```python
from build123d import *

# Parameters (mm, degrees)
F0_W      = 600
F0_H      = 600
F1_DEPTH  = 100
F3_R      = 2
F4_T      = -1.6
F6_DEPTH  = 100.001
F8_DEPTH  = 100.001
F9_R      = 4
F10_DEPTH = 100.001


with BuildPart() as f1:
    # F0 (on Top) → F1 (new body)
    with BuildSketch(Plane.XY):
        Rectangle(F0_W, F0_H)
    extrude(amount=F1_DEPTH)

    # F3
    f3_edges = [f1.edges().sort_by_distance(p)[0] for p in [
        (0, -300, 100),
        (-300, -300, 50),
        (-300, 0, 100),
        (300, -300, 50),
        (-300, 300, 50),
        (300, 0, 100),
        (0, 300, 100),
        (300, 300, 50),
    ]]
    fillet(f3_edges, radius=F3_R)

    # F4
    f4_openings = [f1.faces().sort_by_distance(p)[0] for p in [
        (0, 0, 0),
    ]]
    offset(amount=F4_T, openings=f4_openings)

    # F5 (on face) → F6 (cut, through all)
    with BuildSketch(Plane.XY.offset(100)):
        with BuildLine():
            Line((298, 300), (298, 298))
            Line((298, 298), (300, 298))
            ThreePointArc((300, 298), (299.414214, 299.414214), (298, 300))
        make_face()
        with BuildLine():
            Line((298, -298), (298, -300))
            ThreePointArc((298, -300), (299.414214, -299.414214), (300, -298))
            Line((300, -298), (298, -298))
        make_face()
        with BuildLine():
            Line((-300, 298), (-298, 298))
            Line((-298, 298), (-298, 300))
            ThreePointArc((-298, 300), (-299.414214, 299.414214), (-300, 298))
        make_face()
        with BuildLine():
            ThreePointArc((-300, -298), (-299.414214, -299.414214), (-298, -300))
            Line((-298, -300), (-298, -298))
            Line((-298, -298), (-300, -298))
        make_face()
    extrude(amount=-F6_DEPTH, mode=Mode.SUBTRACT)

    # F7 (on face) → F8 (cut, through all)
    with BuildSketch(Plane.XY.offset(100)):
        with BuildLine():
            ThreePointArc((-20.5, -9.5), (-17.278175, -17.278175), (-9.5, -20.5))
            Line((-9.5, -20.5), (9.5, -20.5))
            ThreePointArc((9.5, -20.5), (17.278175, -17.278175), (20.5, -9.5))
            Line((20.5, -9.5), (20.5, 9.5))
            ThreePointArc((20.5, 9.5), (17.278175, 17.278175), (9.5, 20.5))
            Line((9.5, 20.5), (-9.5, 20.5))
            ThreePointArc((-9.5, 20.5), (-17.278175, 17.278175), (-20.5, 9.5))
            Line((-20.5, 9.5), (-20.5, -9.5))
        make_face()
    extrude(amount=-F8_DEPTH, mode=Mode.SUBTRACT)

    # F9 (on face) → F10 (cut, through all)
    with BuildSketch(Plane.XY.offset(100)):
        with Locations((260, 287)):
            Circle(F9_R)
        with Locations((-260, 287)):
            Circle(F9_R)
        with Locations((-287, -260)):
            Circle(F9_R)
        with Locations((-287, 260)):
            Circle(F9_R)
        with Locations((260, -287)):
            Circle(F9_R)
        with Locations((-260, -287)):
            Circle(F9_R)
        with Locations((287, 260)):
            Circle(F9_R)
        with Locations((287, -260)):
            Circle(F9_R)
    extrude(amount=-F10_DEPTH, mode=Mode.SUBTRACT)


solid = f1.part
```
Input: part model. Units: mm. Frame: model coordinates. A direction names the side the tool comes from. Round coordinates to 2 decimals unless told otherwise and drop trailing zeros. Order: outer loops, then holes, each group sorted by start corner. A loop starts at its lowest first (then second) coordinate and runs counter-clockwise, first axis right, second up. Notation, with made-up numbers: (82.5, -34.5) - (108.5, -34.5) arc R5 cw to (108.5, -27.5) - close; hole circle Ø6 at (-23, 34). An arc over 180 degrees is marked (long way). One line per question, with ' | ' between items. Start each with the question number.
1) Contact query for flat-ended pins moving along their axis: P1, Ø5, axis at x = -43.5, y = 59, coming from the -Z side; P2, Ø1.8, axis at y = -1, z = 99, coming from the -X side; P3, Ø1.6, axis at x = -299, z = 27, coming from the +Y side. Output: stop coordinate, or through.
2) Set-up query: faces 1 (the flat face through (-4, 70, 98.4)), 2 (the flat face through (-300, -4, 48)). Return all of +Z, -Z, +X, -X, +Y, -Y with unobstructed straight access to the full face (end or side cutting, diameter ignored); none if empty.
3) Ray query, probe 1 along Y at (x, z) = (233, 50); probe 2 along X at (y, z) = (-260, 99.15). Return the intervals inside material, ascending.
4) Cut plane A-A, the plane z = 57.5. Return the cut outline in (x, y), then the cut area to 3 significant figures.
5) Pull-direction query (X, two-part tool) for faces 3 (the flat face through (300, -4, 48)), 4 (the flat face through (298.4, -4, 48)), 5 (the flat face through (-4, 300, 48)); classes: +X half, -X half, draft (parallel to the pull), parting line (faces both ways), or undercut.
6) Cut plane B-B, the plane y = 142. Return the cut outline in (x, z).
Worked out:
1) P1: stops at z = 98.4 | P2: stops at x = -300 | P3: stops at y = 298
2) face 1: -Z | face 2: +Z, -Z, -X, +Y, -Y
3) probe 1: y = -300 to -298.4, 298.4 to 300 | probe 2: x = -299.64 to -291, -283 to 283, 291 to 299.64
4) outline: (-300, -298) - (-298.4, -298) - (-298.4, 298) - (-300, 298) - close; (-298, -300) - (298, -300) - (298, -298.4) - (-298, -298.4) - close; (-298, 298.4) - (298, 298.4) - (298, 300) - (-298, 300) - close; (298.4, -298) - (300, -298) - (300, 298) - (298.4, 298) - close | area: 3,810 mm^2
5) face 3: +X half | face 4: undercut | face 5: draft
6) outline: (-300, 0) - (-298.4, 0) - (-298.4, 98) arc R0.4 cw to (-298, 98.4) - (298, 98.4) arc R0.4 cw to (298.4, 98) - (298.4, 0) - (300, 0) - (300, 98) arc R2 ccw to (298, 100) - (-298, 100) arc R2 ccw to (-300, 98) - close
